Drawing for the job (mm, zero at the part's lowest x, y, z). A direction names the side the tool comes from. Give positions to 0.01 mm unless a question says otherwise; leave off trailing zeros. Order: outer loops, then holes, each group sorted by start corner. A loop starts at its lowest first (then second) coordinate and runs counter-clockwise, first axis right, second up. Notation, with made-up numbers: (4.25, -30.75) - (59.25, -30.75) arc R26 cw to (59.25, 5.25) - close; hole circle Ø5 at (-9, -21). An arc over 180 degrees is marked (long way). Use a Markdown table: item, result.
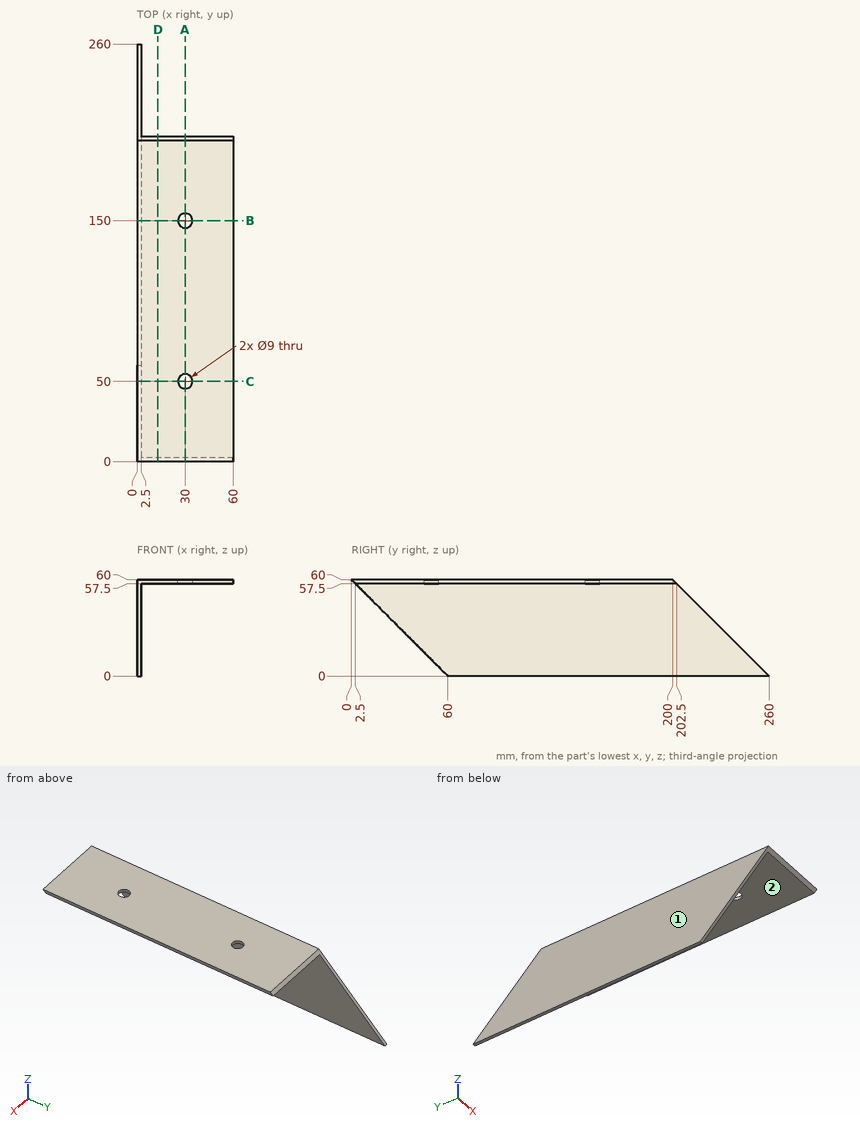
1) Slice it at A-A (x = 30). Write the cut outline in (y, z), and give its area (3 significant figures).
Computed:
| item | result |
|---|---|
| outline | (0, 60) - (2.5, 57.5) - (45.5, 57.5) - (45.5, 60) - close; (54.5, 57.5) - (145.5, 57.5) - (145.5, 60) - (54.5, 60) - close; (154.5, 57.5) - (202.5, 57.5) - (200, 60) - (154.5, 60) - close |
| area | 455 mm² |
2) Slice it at D-D (x = 13). Write the cut outline in (y, z), and give its area (3 significant figures).
Computed:
| item | result |
|---|---|
| outline | (0, 60) - (2.5, 57.5) - (202.5, 57.5) - (200, 60) - close |
| area | 500 mm² |
3) Wall check: line 1 (X direction, y = 50, z = 58); line 2 (Y direction, x = 30, z = 58.25); line 3 (X direction, y = 222, z = 17.5). Give the ranges that are in metal, low to high. Write a range as from..to.
Computed:
| item | result |
|---|---|
| line 1 | x = 0..25.5, 34.5..60 |
| line 2 | y = 1.75..45.5, 54.5..145.5, 154.5..201.75 |
| line 3 | x = 0..2.5 |
4) Tool access for the marked faces 1 and 2: list every direction of +Z, -Z, +X, -X, +Y, -Y with a clear straight run to the whole face (end or side of a thin tool).
Computed:
| item | result |
|---|---|
| face 1 | +Z, -Z, -X, +Y, -Y |
| face 2 | -Z, +X, +Y, -Y |
5) Slice it at C-C (y = 50). Write the cut outline in (x, z), and give its area (3 significant figures).
Computed:
| item | result |
|---|---|
| outline | (0, 10) - (2.5, 10) - (2.5, 57.5) - (25.5, 57.5) - (25.5, 60) - (0, 60) - close; (34.5, 57.5) - (60, 57.5) - (60, 60) - (34.5, 60) - close |
| area | 246 mm² |
6) Pin check, flat tips, straight feed: P1, Ø2, axis at x = 47, y = 106.5, coming from the -Z side; P2, Ø2, axis at y = 75, z = 52, coming from the +X side; P3, Ø8, axis at x = 30, y = 50, coming from the +Z side. Stop position of each tip, or through.
Computed:
| item | result |
|---|---|
| P1 | stops at z = 57.5 |
| P2 | stops at x = 2.5 |
| P3 | passes through |
7) Slice it at B-B (y = 150). Write the cut outline in (x, z).
Computed:
| item | result |
|---|---|
| outline | (0, 0) - (2.5, 0) - (2.5, 57.5) - (25.5, 57.5) - (25.5, 60) - (0, 60) - close; (34.5, 57.5) - (60, 57.5) - (60, 60) - (34.5, 60) - close |
